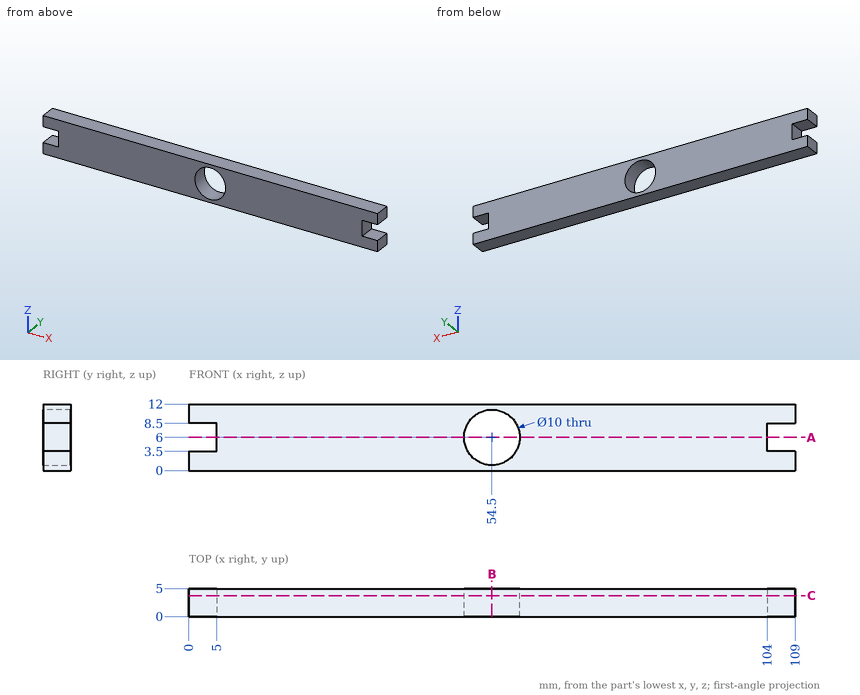
Part print with two shaded views. Sizes in mm from the minimum x, y, z corner. Give positions to 0.01 mm unless a question says otherwise; leave off trailing zeros. Order: outer loops, then holes, each group sorted by start corner. A loop starts at its lowest first (then second) coordinate and runs counter-clockwise, first axis right, second up.
(1) Drill centre lines: L1, parallel to X at y = 0.7, z = 6; L2, parallel to X at y = 1.9, z = 10.5. Where is each one in solid material? Low to high.
(2) Saw through at C-C, the plane y = 3.75. Give the cut face in (x, z), then the cut area to 3 significant figures.
(3) Flat gauge pins, fed straight in: pin 1 (2.5 mm diameter, centred on y = 2, z = 6.5, fed in from -X); pin 2 (2.5 mm diameter, centred on y = 1.5, z = 5, fed in from +X). Where does each tip first touch, or does it go through?
(4) Saw through at A-A, the plane z = 6. Give the cut face in (x, y).
(5) Saw through at B-B, the plane x = 54.5. Give the cut face in (y, z), then the cut area to 3 significant figures.
Results found:
1. L1: x = 5 to 49.5, 59.5 to 104
1. L2: x = 0 to 52.32, 56.68 to 109
2. outline: (0, 0) - (109, 0) - (109, 3.5) - (104, 3.5) - (104, 8.5) - (109, 8.5) - (109, 12) - (0, 12) - (0, 8.5) - (5, 8.5) - (5, 3.5) - (0, 3.5) - close; hole circle Ø10 at (54.5, 6)
2. area: 1,180 mm2
3. pin 1: stops at x = 5
3. pin 2: stops at x = 104
4. outline: (5, 0) - (49.5, 0) - (49.5, 5) - (5, 5) - close; (59.5, 0) - (104, 0) - (104, 5) - (59.5, 5) - close
5. outline: (0, 0) - (5, 0) - (5, 1) - (0, 1) - close; (0, 11) - (5, 11) - (5, 12) - (0, 12) - close
5. area: 10.0 mm2
